Could you check a few things on this model? Use its own coordinates, in mm. Coordinates: 2 decimals unless noted, no trailing zeros. Loops run counter-clockwise (first coordinate to the right, second up) from the corner with the lowest first, then second, coordinate; pieces in that order, holes last. Notation, with made-up numbers: M 27.25,40 L 63.25,40 A21 cw 63.25,63 Z; hole C 15,-36.75 d11. An arc over 180 degrees is marked long. Write each question's results on one line, items separated by ' | '.
```python
from build123d import *

# Parameters (mm, degrees)
SKETCH1_W                    = 130
SKETCH1_H                    = 30
SKETCH1_R                    = 2
BASE_FLANGE1_DEPTH           = 0.7366
EDGE_FLANGE1_STRIP_W         = 4.4196
EDGE_FLANGE1_STRIP_H         = 0.7366
EDGE_FLANGE1_STRIP_CUT_DEPTH = 130
EDGE_FLANGE1_DEPTH           = 130


# Sheet-metal steps are written as plain solids
with BuildPart() as part:
    # Sketch1 → Base-Flange1 (new body)
    with BuildSketch(Plane(origin=(0, 0, 0), x_dir=(1, 0, 0), z_dir=(0, 1, 0))):
        Rectangle(SKETCH1_W, SKETCH1_H)
        with Locations(Location((0, 5, 0), (0, 0, 270))):
            Circle(SKETCH1_R, mode=Mode.SUBTRACT)
        with Locations(Location((-21.666666667, -5, 0), (0, 0, 270))):
            Circle(SKETCH1_R, mode=Mode.SUBTRACT)
        with Locations(Location((-43.333333333, 5, 0), (0, 0, 270))):
            Circle(SKETCH1_R, mode=Mode.SUBTRACT)
        with Locations(Location((21.666666667, -5, 0), (0, 0, 270))):
            Circle(SKETCH1_R, mode=Mode.SUBTRACT)
        with Locations(Location((43.333333333, 5, 0), (0, 0, 270))):
            Circle(SKETCH1_R, mode=Mode.SUBTRACT)
    extrude(amount=-BASE_FLANGE1_DEPTH)

    # Edge-Flange1 strip (across the edge) → Edge-Flange1 strip cut (cut)
    with BuildSketch(Plane(origin=(65, 0, -15), x_dir=(0, 0, 1), z_dir=(-1, 0, 0))):
        with Locations((-0.7366, -0.3683)):
            Rectangle(EDGE_FLANGE1_STRIP_W, EDGE_FLANGE1_STRIP_H)
    extrude(amount=EDGE_FLANGE1_STRIP_CUT_DEPTH, mode=Mode.SUBTRACT)

    # Edge-Flange1 section (across the edge) → Edge-Flange1 (add)
    with BuildSketch(Plane(origin=(65, 0, -15), x_dir=(0, 0, 1), z_dir=(-1, 0, 0))):
        with BuildLine():
            Line((0, 0.7366), (0, 29.6534))
            Line((0, 29.6534), (0.7366, 29.6534))
            Line((0.7366, 29.6534), (0.7366, 0.7366))
            ThreePointArc((0.7366, 0.7366), (0.952345145, 0.215745145), (1.4732, 0))
            Line((1.4732, 0), (1.4732, -0.7366))
            ThreePointArc((1.4732, -0.7366), (0.43149029, -0.30510971), (0, 0.7366))
        make_face()
    extrude(amount=EDGE_FLANGE1_DEPTH)


solid = part.part
```
(1) If we mould it in two halves opening along Z, with no side actions, what happens to faces 1 (the flat face through (1, 15, -14.263)), 2 (the cylindrical face through (-41.35, -0.36, -5.26)), 3 (the flat face through (-1, 0, 1))? For each: released by +Z, released by -Z, zero draft, split by the parting line, or undercut.
Reported:
face 1: released by +Z | face 2: undercut | face 3: zero draft
(2) Imagine slicing it at A-A, the plane z = -5. List the corners of the cut face in (x, y) for me, and give its area (3 significant figures).
Reported:
outline: M -65,-0.74 L -45.33,-0.74 L -45.33,0 L -65,0 Z; M -41.33,-0.74 L -2,-0.74 L -2,0 L -41.33,0 Z; M 2,-0.74 L 41.33,-0.74 L 41.33,0 L 2,0 Z; M 45.33,-0.74 L 65,-0.74 L 65,0 L 45.33,0 Z | area: 86.9 mm2
(3) Imagine slicing it at B-B, the plane x = 0. List the corners of the cut face in (y, z) for me, and give its area (3 significant figures).
Reported:
outline: M -0.74,-13.53 A1.47 ccw 0.74,-15 L 29.65,-15 L 29.65,-14.26 L 0.74,-14.26 A0.74 cw 0,-13.53 L 0,-7 L -0.74,-7 Z; M -0.74,-3 L 0,-3 L 0,15 L -0.74,15 Z | area: 40.6 mm2
(4) Please list where these lines run through material, in increasing order: probe 1 along X at (y, z) = (-0.5, -5); probe 2 along X at (y, z) = (-0.5, 5); probe 3 along Z at (x, y) = (-20, 20). Write a range as from..to.
Reported:
probe 1: x = -65..-45.33, -41.33..-2, 2..41.33, 45.33..65 | probe 2: x = -65..-23.67, -19.67..19.67, 23.67..65 | probe 3: z = -15..-14.26
(5) Will these pins go through, and if not, where does the flat tip stop? P1, Ø2, axis at x = -12, y = 13.5, coming from the +Z side; P2, Ø6.5, axis at x = 43.33, z = -5, coming from the -Y side; P3, Ø4.5, axis at x = 0, z = -5, coming from the +Y side.
Reported:
P1: stops at z = -14.26 | P2: stops at y = -0.74 | P3: stops at y = 0
(6) Imagine slicing it at D-D, the plane x = 38.5. List the corners of the cut face in (y, z) for me.
Reported:
outline: M -0.74,-13.53 A1.47 ccw 0.74,-15 L 29.65,-15 L 29.65,-14.26 L 0.74,-14.26 A0.74 cw 0,-13.53 L 0,15 L -0.74,15 Z
(7) Imagine slicing it at C-C, the plane z = 5. List the corners of the cut face in (x, y) for me, and give its area (3 significant figures).
Reported:
outline: M -65,-0.74 L -23.67,-0.74 L -23.67,0 L -65,0 Z; M -19.67,-0.74 L 19.67,-0.74 L 19.67,0 L -19.67,0 Z; M 23.67,-0.74 L 65,-0.74 L 65,0 L 23.67,0 Z | area: 89.9 mm2
